The model under review builds one solid part; all positions refer to its coordinate system, in mm. A direction names the side the tool comes from. Round coordinates to 2 decimals unless told otherwise and drop trailing zeros. Order: outer loops, then holes, each group sorted by start corner. A loop starts at its lowest first (then second) coordinate and runs counter-clockwise, first axis right, second up. Notation, with made-up numbers: (44.25, -22.5) -> (54.25, -22.5) arc R23 ccw to (54.25, -11.5) -> close; hole circle Ø9 at (-21.75, 65). An arc over 180 degrees is marked (long way). Use a Markdown table: item, result. Add a question column.
```python
from build123d import *

# Parameters (mm, degrees)
PAD_DEPTH       = 3
SKETCH001_W     = 78
SKETCH001_H     = 71
PAD001_DEPTH    = 3
CHAMFER_SIZE    = 3
SKETCH002_W     = 74
SKETCH002_H     = 67
POCKET_DEPTH    = 3
CHAMFER001_SIZE = 2
SKETCH003_R     = 4
SKETCH003_R_2   = 1.5
PAD002_DEPTH    = 18


with BuildPart() as part:
    # Sketch → Pad (new body)
    with BuildSketch(Plane.XY):
        Polygon((38.5, 39), (-38.5, 39), (-42.5, 35), (-42.5, -35), (-38.5, -39), (38.5, -39), (42.5, -35), (42.5, 35), align=None)
    extrude(amount=PAD_DEPTH)

    # Sketch001 (on Face9 of Pad) → Pad001 (join)
    with BuildSketch(Plane(origin=(0, 0, 0), x_dir=(1, 0, 0), z_dir=(0, 0, -1))):
        Rectangle(SKETCH001_W, SKETCH001_H)
    extrude(amount=PAD001_DEPTH)

    # Chamfer
    chamfer_edges = [part.edges().sort_by_distance(p)[0] for p in [
        (39, 35.5, -1.5),
        (-39, 35.5, -1.5),
        (-39, -35.5, -1.5),
        (39, -35.5, -1.5),
    ]]
    chamfer(chamfer_edges, length=CHAMFER_SIZE)

    # Sketch002 (on Face18 of Chamfer) → Pocket (cut)
    with BuildSketch(Plane(origin=(0, 0, -3), x_dir=(1, 0, 0), z_dir=(0, 0, -1))):
        Rectangle(SKETCH002_W, SKETCH002_H)
    extrude(amount=-POCKET_DEPTH, mode=Mode.SUBTRACT)

    # Chamfer001
    chamfer001_edges = [part.edges().sort_by_distance(p)[0] for p in [
        (37, 33.5, -1.5),
        (-37, 33.5, -1.5),
        (-37, -33.5, -1.5),
        (37, -33.5, -1.5),
    ]]
    chamfer(chamfer001_edges, length=CHAMFER001_SIZE)

    # Sketch003 (on Face18 of Chamfer001) → Pad002 (join)
    with BuildSketch(Plane(origin=(0, 0, 0), x_dir=(1, 0, 0), z_dir=(0, 0, -1))):
        with Locations((-30.7975, 28.01)):
            Circle(SKETCH003_R)
        with Locations((-30.7975, 28.01)):
            Circle(SKETCH003_R_2, mode=Mode.SUBTRACT)
        with Locations((30.7975, 28.01)):
            Circle(SKETCH003_R)
        with Locations((30.7975, 28.01)):
            Circle(SKETCH003_R_2, mode=Mode.SUBTRACT)
        with Locations((-30.7975, -31.045)):
            Circle(SKETCH003_R)
        with Locations((-30.7975, -31.045)):
            Circle(SKETCH003_R_2, mode=Mode.SUBTRACT)
        with Locations((30.7975, -31.045)):
            Circle(SKETCH003_R)
        with Locations((30.7975, -31.045)):
            Circle(SKETCH003_R_2, mode=Mode.SUBTRACT)
    extrude(amount=PAD002_DEPTH)


solid = part.part
```
Q1. Add section A-A (z = -7.5). Write out the cut boundary in (x, y) (1 decimal).
Q2. Insertion check: pin 1 (2.5 mm diameter, centred on y = -4.5, z = -2, fed in from -X); pin 2 (1.5 mm diameter, centred on y = -0.5, z = -2, fed in from +X); pin 3 (23.5 mm diameter, centred on x = -21, y = -1.5, fed in from -Z); pin 4 (6 mm diameter, centred on y = 13.5, z = -7.5, fed in from +X). Each pin has a flat end and moves straight along its axis. Give the tip position at first contact, or say it passes through.
Q3. Add section B-B (y = -2.5). Write out the cut boundary in (x, z).
Q4. Machinability: for faces 1 (the flat face through (39, 0, -1)), 2 (the flat face through (-42.5, 0, 1)), 3 (the flat face through (-31, 31, 0)), 4 (the flat face through (37.5, -34, -1.5)), which of the approach directions +Z, -Z, +X, -X, +Y, -Y give a long, thin tool a straight path to every point of the face, cutting with its end or side? Answer none if there is none.
Q5. Add section C-C (x = 4). Write out the cut boundary in (y, z), then the cut area to 3 significant figures.
Q6. Mouldability with a two-part tool opening along Y and no side actions: class faces 5 (the flat face through (-31, 33, -18)), 6 (the flat face through (-1, 35.5, -1)), 7 (the flat face through (-1, 0, 0)) as pulls with the +Y half, pulls with the -Y half, needs draft (parallel to the pull), parting line crosses it, or undercut.
Q7. Wall thickness on line 1 (X direction, y = -28.01, z = -3.5); line 2 (Y direction, x = -9, z = -2); line 3 (Y direction, x = 31, z = -14.5): over which ranges is each line inside the solid? List them lowest first. Write a range as [from, to].
Q8. Add section D-D (y = -28.01). Write out the cut boundary in (x, z), then the cut area to 3 significant figures.
Report:
| question | item | result |
|---|---|---|
| 1 | outline | circle Ø8 at (-30.8, -28); circle Ø8 at (-30.8, 31); circle Ø8 at (30.8, -28); circle Ø8 at (30.8, 31); hole circle Ø3 at (-30.8, -28); hole circle Ø3 at (-30.8, 31); hole circle Ø3 at (30.8, -28); hole circle Ø3 at (30.8, 31) |
| 2 | pin 1 | stops at x = -39 |
| 2 | pin 2 | stops at x = 39 |
| 2 | pin 3 | stops at z = 0 |
| 2 | pin 4 | passes through |
| 3 | outline | (-42.5, 0) -> (-39, 0) -> (-39, -3) -> (-37, -3) -> (-37, 0) -> (37, 0) -> (37, -3) -> (39, -3) -> (39, 0) -> (42.5, 0) -> (42.5, 3) -> (-42.5, 3) -> close |
| 4 | face 1 | -Z, +X, +Y, -Y |
| 4 | face 2 | +Z, -Z, -X, +Y, -Y |
| 4 | face 3 | -Z |
| 4 | face 4 | -Z, +X, -Y |
| 5 | outline | (-39, 0) -> (-35.5, 0) -> (-35.5, -3) -> (-33.5, -3) -> (-33.5, 0) -> (33.5, 0) -> (33.5, -3) -> (35.5, -3) -> (35.5, 0) -> (39, 0) -> (39, 3) -> (-39, 3) -> close |
| 5 | area | 246 mm² |
| 6 | face 5 | needs draft |
| 6 | face 6 | pulls with the +Y half |
| 6 | face 7 | undercut |
| 7 | line 1 | x = [-34.8, -32.3], [-29.3, -26.8], [26.8, 29.3], [32.3, 34.8] |
| 7 | line 2 | y = [-35.5, -33.5], [33.5, 35.5] |
| 7 | line 3 | y = [-32, -29.5], [-26.52, -24.02], [27.05, 29.56], [32.53, 35.04] |
| 8 | outline | (-42.5, 0) -> (-39, 0) -> (-39, -3) -> (-37, -3) -> (-37, 0) -> (-34.8, 0) -> (-34.8, -18) -> (-32.3, -18) -> (-32.3, 0) -> (-29.3, 0) -> (-29.3, -18) -> (-26.8, -18) -> (-26.8, 0) -> (26.8, 0) -> (26.8, -18) -> (29.3, -18) -> (29.3, 0) -> (32.3, 0) -> (32.3, -18) -> (34.8, -18) -> (34.8, 0) -> (37, 0) -> (37, -3) -> (39, -3) -> (39, 0) -> (42.5, 0) -> (42.5, 3) -> (-42.5, 3) -> close |
| 8 | area | 447 mm² |
